Autodesk Inventor part; units mm, degrees
ref_plane "YZ Plane" through (0, 0, 0) normal (1, 0, 0) x (0, 1, 0)
ref_plane "XZ Plane" through (0, 0, 0) normal (0, 1, 0) x (-1, 0, 0)
ref_plane "XY Plane" through (0, 0, 0) normal (0, 0, 1) x (1, 0, 0)
sketch "Sketch1" plane through (0, 0, 0) normal (0, 0, 1) x (1, 0, 0)
  line L0 (-55.88, -28.575) -> (55.88, -28.575)
  line L1 (55.88, -28.575) -> (55.88, 28.575)
  line L2 (55.88, 28.575) -> (-55.88, 28.575)
  line L3 (-55.88, 28.575) -> (-55.88, -28.575)
  line L4 (-55.88, -28.575) -> (55.88, 28.575) construction
  line L5 (55.88, -28.575) -> (-55.88, 28.575) construction
  circle A0 centre (-52.07, 24.765) radius 1.4
  line L6 (-55.88, 0) -> (55.88, 0) construction
  line L7 (0, 28.575) -> (0, -28.575) construction
  circle A1 centre (-52.07, -24.765) radius 1.4
  circle A2 centre (-31.75, 24.765) radius 1.4
  circle A3 centre (31.75, 24.765) radius 1.4
  circle A4 centre (-31.75, -24.765) radius 1.4
  circle A5 centre (31.75, -24.765) radius 1.4
  circle A6 centre (50.8, 25.865) radius 0.99
  circle A7 centre (41.91, 24.765) radius 1.4
  circle A8 centre (41.91, -24.765) radius 1.4
  circle A9 centre (50.8, -2.71) radius 0.8
  point P0 (0, 0)
  dimension "d2" = 111.76
  dimension "d4" = 57.15
  dimension "d5" = 49.53
  dimension "d6" = 2.8
  dimension "d8" = 2.8
  dimension "d10" = 49.53
  dimension "d21" = 3.81
  dimension "d22" = 3.81
  dimension "d23" = 3.81
  dimension "d28" = 3.81
  dimension "d30" = 63.5
  dimension "d35" = 1.98
  dimension "d36" = 5.08
  dimension "d37" = 2.71
  dimension "d38" = 2.8
  dimension "d39" = 3.81
  dimension "d40" = 13.97
  dimension "d41" = 63.5
  dimension "d42" = 1.6
  dimension "d43" = 5.08
  dimension "d44" = 2.71
extrude "Extrusion1" add sketch "Sketch1" along normal blind 1.6 contours L3 L2 L1 L0 | A2 | A3 | A4 | A5
sketch "Sketch3" plane through (0, 0, 1.6) normal (0, 0, 1) x (1, 0, 0)
  circle A0 centre (26.67, -24.765) radius 1.4
  circle A1 centre (-26.67, -24.765) radius 1.4
  line L0 (55.88, 28.575) -> (-55.88, 28.575)
  line L1 (-21.67, -25.765) -> (21.67, -25.765)
  line L2 (21.67, -25.765) -> (21.67, 30.575)
  line L3 (21.67, 30.575) -> (-21.67, 30.575)
  line L4 (-21.67, 30.575) -> (-21.67, -25.765)
  line L5 (55.88, -28.575) -> (55.88, 28.575)
  line L6 (-55.88, 28.575) -> (-55.88, -28.575)
  point P0 (0, 0)
  dimension "d15" = 2
  dimension "d16" = 5
  dimension "d17" = 5
  dimension "d18" = 1
  dimension "d33" = 34.21
  dimension "d34" = 34.21
extrude "Extrusion3" [suppressed]
properties part number "BetaBoard01" material "PCB(1)"
Geometry: final body of the model. Coordinates: model frame, mm. Coordinates: 2 decimals unless noted, no trailing zeros. Order: outer loops, then holes, each group sorted by start corner. A loop starts at its lowest first (then second) coordinate and runs counter-clockwise, first axis right, second up. Notation, with made-up numbers: M -17.5,18.25 L 35.5,18.25 A17 ccw 35.5,50.25 Z; hole C 69.5,44 d10. An arc over 180 degrees is marked long. Answer in a Markdown table with one row per item. Add a question column.
Q1. Line query: L1, parallel to Y at x = -52.07, z = 1.3 (3 decimals); L2, parallel to Y at x = 50.8, z = 0.85 (3 decimals); L3, parallel to X at y = 25, z = 0.15. Output: solid intervals per line, ascending.
Q2. Mould query, pull axis X, two halves, no side actions, for faces 1 (the cylindrical face through (49.81, 25.82, 0.79)), 2 (the flat face through (-1, 0, 1.6)). Classes: released by +X, released by -X, zero draft, split by the parting line, or undercut.
Q3. Section query A-A on x = 41.91. Return the cut outline in (y, z) (3 decimals).
Completed:
| question | item | result |
|---|---|---|
| 1 | L1 | y = -28.575 to -26.165, -23.365 to 23.365, 26.165 to 28.575 |
| 1 | L2 | y = -28.575 to -3.51, -1.91 to 24.875, 26.855 to 28.575 |
| 1 | L3 | x = -55.88 to -53.45, -50.69 to 40.53, 43.29 to 50.32, 51.28 to 55.88 |
| 2 | face 1 | undercut |
| 2 | face 2 | zero draft |
| 3 | outline | M -28.575,0 L -26.165,0 L -26.165,1.6 L -28.575,1.6 Z; M -23.365,0 L 23.365,0 L 23.365,1.6 L -23.365,1.6 Z; M 26.165,0 L 28.575,0 L 28.575,1.6 L 26.165,1.6 Z |
